Check sheet for the modelled part. Datum: model origin and axes. Units: mm. Face numbers are marked on the shaded views. A direction names the side the tool comes from. Give positions to 0.01 mm unless a question says otherwise; leave off trailing zeros. Order: outer loops, then holes, each group sorted by start corner. A loop starts at its lowest first (then second) coordinate and runs counter-clockwise, first axis right, second up.
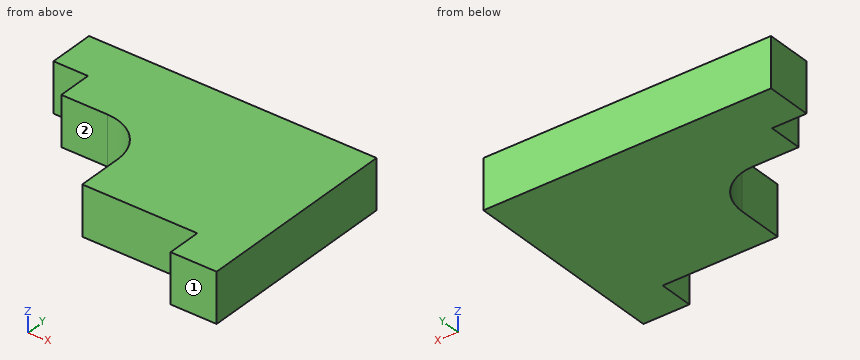
from build123d import *

# Parameters (mm, degrees)
BOSS_EXTRUDE1_DEPTH = 21.542835


with BuildPart() as part:
    # Sketch1 → Boss-Extrude1 (new body)
    with BuildSketch(Plane.XY):
        with BuildLine():
            Line((150, 110), (150, 130))
            ThreePointArc((150, 130), (144.142135624, 144.142135624), (130, 150))
            Line((130, 150), (110, 150))
            Line((110, 150), (110, 165))
            Line((110, 165), (95, 165))
            Line((95, 165), (95, 185))
            Line((95, 185), (220, 185))
            Line((220, 185), (220, 95))
            Line((220, 95), (200, 95))
            Line((200, 95), (200, 110))
            Line((200, 110), (150, 110))
        make_face()
    extrude(amount=-BOSS_EXTRUDE1_DEPTH)


solid = part.part
1) Set-up check for the marked faces 1 and 2: record each of +Z, -Z, +X, -X, +Y, -Y from which the full face is reachable in a straight line by a thin tool's end or side.
Recorded:
face 1: +Z, -Z, +X, -X, -Y
face 2: +Z, -Z, -X, -Y
2) Section check C-C, the plane x = 190.5. Record the cut outline in (y, z).
Recorded:
outline: (110, -21.54) - (185, -21.54) - (185, 0) - (110, 0) - close
3) Section check A-A, the plane z = -17. Record the cut outline in (x, y), then the cut area to 3 significant figures.
Recorded:
outline: (95, 165) - (110, 165) - (110, 150) - (130, 150) arc R20 cw to (150, 130) - (150, 110) - (200, 110) - (200, 95) - (220, 95) - (220, 185) - (95, 185) - close
area: 7,340 mm2
4) Material ranges on L1, parallel to X at y = 150.5, z = -12.75; L2, parallel to X at y = 127.5, z = -11.5; L3, parallel to Y at x = 187, z = -10, recorded low to high.
Recorded:
L1: x = 110 to 220
L2: x = 150 to 220
L3: y = 110 to 185
5) Section check B-B, the plane y = 154.5. Record the cut outline in (x, z).
Recorded:
outline: (110, -21.54) - (220, -21.54) - (220, 0) - (110, 0) - close
6) Depth check by flat-ended pin: pin 1 Ø4 at (y, z) = (149, -3.5) entering from -X; pin 2 Ø5 at (x, z) = (140, -11) entering from -Y; pin 3 Ø12 at (y, z) = (99, -9.5) entering from -X. Enter the tip coordinate at first touch or a pass-through.
Recorded:
pin 1: stops at x = 110
pin 2: stops at y = 145.61
pin 3: stops at x = 200
